Here's how the part is built. I have some questions about the finished solid (model axes, mm). Round coordinates to 2 decimals unless told otherwise and drop trailing zeros. Write each loop counter-clockwise with the first axis right and the second up, starting at its lowest first coordinate (ties: lowest second). Pieces come first, ordered by that corner, then holes. Notation, with made-up numbers: M 35.25,14.25 L 86.25,14.25 A32 cw 86.25,45.25 Z; hole C 23,74 d10. An arc over 180 degrees is marked long. Write item = value, one per line. Start each with the question number.
(1) If we mould it in two halves opening along Z, with no side actions, what happens to faces 1 (the flat face through (12.37, 2.46, -29.88)), 2 (the cylindrical face through (-10.148, 2.465, -21.393)), 3 (the flat face through (0, 0, 2))? For each: released by +Z, released by -Z, zero draft, split by the parting line, or undercut.
(2) I want a section at A-A (x = -19). List the corners of the cut face in (y, z) for me.
(3) Will these pins go through, and if not, where does the flat tip stop? pin 1 Ø3.5 at (x, z) = (-19.92, -11.5) entering from -Y; pin 2 Ø1 at (y, z) = (1.5, -18) entering from +X.
(4) I want a section at C-C (y = 3). Give the number of separate pieces and of enclosed holes in the cut face, and give its area (3 significant figures).
(5) I need wall thicknesses on line 1 along X through (y, z) = (3.3, 0); line 2 along Z through (x, y) = (-13, 3.15); line 3 along X through (y, z) = (3.7, 11.5). Which ranges of each line are inside material? Lowest first, please.
(6) I want a section at B-B (z = 11.5). List the corners of the cut face in (x, y) for me, and give its area (3 significant figures).
(7) I want a section at D-D (z = -23). List the corners of the cut face in (x, y) for me.
```python
from build123d import *

# Parameters (mm, degrees)
SKETCH1_R           = 30
SKETCH1_R_2         = 2
SKETCH1_R_3         = 5
SKETCH1_R_4         = 2.5
BOSS_EXTRUDE1_DEPTH = 5


with BuildPart() as part:
    # Sketch1 → Boss-Extrude1 (new body)
    # profile 1 of 4: a face of its own
    with BuildSketch(Plane(origin=(0, 0, 0), x_dir=(1, 0, 0), z_dir=(0, 1, 0))):
        Circle(SKETCH1_R)
        with Locations(Location((-11.5, 19.918584287, 0), (0, 0, 270))):
            Circle(SKETCH1_R_2, mode=Mode.SUBTRACT)
        with Locations(Location((-19.918584287, 11.5, 0), (0, 0, 270))):
            Circle(SKETCH1_R_2, mode=Mode.SUBTRACT)
        with Locations(Location((-23, 0, 0), (0, 0, 270))):
            Circle(SKETCH1_R_2, mode=Mode.SUBTRACT)
        with Locations(Location((-19.918584287, -11.5, 0), (0, 0, 270))):
            Circle(SKETCH1_R_2, mode=Mode.SUBTRACT)
        with Locations(Location((-11.5, -19.918584287, 0), (0, 0, 270))):
            Circle(SKETCH1_R_2, mode=Mode.SUBTRACT)
        with Locations(Location((0, -23, 0), (0, 0, 270))):
            Circle(SKETCH1_R_2, mode=Mode.SUBTRACT)
        with Locations(Location((11.5, -19.918584287, 0), (0, 0, 270))):
            Circle(SKETCH1_R_2, mode=Mode.SUBTRACT)
        with Locations(Location((19.918584287, -11.5, 0), (0, 0, 270))):
            Circle(SKETCH1_R_2, mode=Mode.SUBTRACT)
        with Locations(Location((23, 0, 0), (0, 0, 270))):
            Circle(SKETCH1_R_2, mode=Mode.SUBTRACT)
        with Locations(Location((19.918584287, 11.5, 0), (0, 0, 270))):
            Circle(SKETCH1_R_2, mode=Mode.SUBTRACT)
        with Locations(Location((11.5, 19.918584287, 0), (0, 0, 270))):
            Circle(SKETCH1_R_2, mode=Mode.SUBTRACT)
        with Locations(Location((0, 23, 0), (0, 0, 270))):
            Circle(SKETCH1_R_2, mode=Mode.SUBTRACT)
    # profile 2 of 4: a face of its own
    with BuildSketch(Plane(origin=(0, 0, 0), x_dir=(1, 0, 0), z_dir=(0, 1, 0))):
        with BuildLine():
            Line((20.995626367, 21.428571429), (3.499271061, 38.571428571))
            ThreePointArc((3.499271061, 38.571428571), (4.609574563, 36.936962144), (5, 35))
            ThreePointArc((5, 35), (3.535533899, 31.464466087), (-1.9e-08, 30))
            ThreePointArc((-1.9e-08, 30), (11.338934182, 27.774602997), (20.995626367, 21.428571429))
        make_face()
    # profile 3 of 4: a face of its own
    with BuildSketch(Plane(origin=(0, 0, 0), x_dir=(1, 0, 0), z_dir=(0, 1, 0))):
        with BuildLine():
            ThreePointArc((-1.9e-08, 30), (-4.629100502, 33.110177644), (-3.499271061, 38.571428571))
            Line((-3.499271061, 38.571428571), (-20.995626367, 21.428571429))
            ThreePointArc((-20.995626367, 21.428571429), (-11.338934199, 27.77460299), (-1.9e-08, 30))
        make_face()
    # profile 4 of 4: a face of its own
    with BuildSketch(Plane(origin=(0, 0, 0), x_dir=(1, 0, 0), z_dir=(0, 1, 0))):
        with Locations((0, 35)):
            Circle(SKETCH1_R_3)
        with Locations(Location((0, 35, 0), (0, 0, 270))):
            Circle(SKETCH1_R_4, mode=Mode.SUBTRACT)
    extrude(amount=BOSS_EXTRUDE1_DEPTH)


solid = part.part
```
Returned:
q1.face_1 = released by -Z
q1.face_2 = undercut
q1.face_3 = zero draft
q2.outline = M 0,-23.38 L 5,-23.38 L 5,-13.28 L 0,-13.28 Z; M 0,-9.72 L 5,-9.72 L 5,9.72 L 0,9.72 Z; M 0,13.28 L 5,13.28 L 5,23.22 L 0,23.22 Z
q3.pin_1 = through
q3.pin_2 = 24.37
q4.separate_pieces = 1
q4.enclosed_holes = 13
q4.area = 2,840 mm²
q5.line_1 = -30 to -25, -21 to 21, 25 to 30
q5.line_2 = -29.26 to -21.24, -18.6 to 18.6, 21.24 to 27.04
q5.line_3 = -27.71 to -21.92, -17.92 to 17.92, 21.92 to 27.71
q6.outline = M -27.71,0 L -21.92,0 L -21.92,5 L -27.71,5 Z; M -17.92,0 L 17.92,0 L 17.92,5 L -17.92,5 Z; M 21.92,0 L 27.71,0 L 27.71,5 L 21.92,5 Z
q6.area = 237 mm²
q7.outline = M -19.39,0 L -2,0 L -2,5 L -19.39,5 Z; M 2,0 L 19.39,0 L 19.39,5 L 2,5 Z
